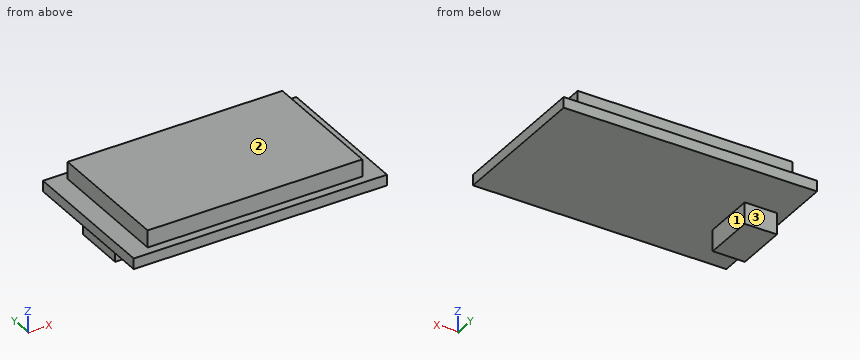
Autodesk Inventor part; units mm, degrees
ref_plane "YZ Plane" through (0, 0, 0) normal (1, 0, 0) x (0, 1, 0)
ref_plane "XZ Plane" through (0, 0, 0) normal (0, 1, 0) x (-1, 0, 0)
ref_plane "XY Plane" through (0, 0, 0) normal (0, 0, 1) x (1, 0, 0)
sketch "Sketch1" plane through (0, 0, 0) normal (0, 0, 1) x (1, 0, 0)
  line L0 (-29.5, -17) -> (29.5, -17)
  line L1 (29.5, -17) -> (29.5, 17)
  line L2 (29.5, 17) -> (-29.5, 17)
  line L3 (-29.5, 17) -> (-29.5, -17)
  line L4 (-29.5, -17) -> (29.5, 17) construction
  line L5 (29.5, -17) -> (-29.5, 17) construction
  point P0 (0, 0)
  dimension "d0" = 59
  dimension "d1" = 34
extrude "Extrusion1" add sketch "Sketch1" along normal blind 2.5
sketch "Sketch2" plane through (0, 0, 2.5) normal (0, 0, 1) x (1, 0, 0)
  line L0 (-25, -15) -> (25, -15)
  line L1 (25, -15) -> (25, 15)
  line L2 (25, 15) -> (-25, 15)
  line L3 (-25, 15) -> (-25, -15)
  line L4 (-25, -15) -> (25, 15) construction
  line L5 (25, -15) -> (-25, 15) construction
  point P0 (0, 0)
  dimension "d4" = 50
  dimension "d5" = 30
extrude "Extrusion2" add sketch "Sketch2" along normal blind 4
sketch "Sketch3" plane through (0, 0, 0) normal (0, 0, -1) x (-1, 0, 0)
  line L0 (-41.3, 0) -> (41.3, 0)
  line L1 (27, 6) -> (19.5, 6)
  line L2 (19.5, 6) -> (19.5, -6)
  line L3 (19.5, -6) -> (27, -6)
  line L4 (27, -6) -> (27, 6)
  line L5 (27, 6) -> (19.5, -6) construction
  line L6 (19.5, 6) -> (27, -6) construction
  line L7 (29.5, 17) -> (29.5, -17)
  point P0 (0, 0)
  point P1 (23.25, 0)
  dimension "d8" = 7.5
  dimension "d9" = 12
  dimension "d10" = 2.5
extrude "Extrusion3" add sketch "Sketch3" along normal blind 5
properties part number "lcdsw"
The model under review builds one solid part; all positions refer to its coordinate system, in mm. Face numbers are marked on the shaded views. A direction names the side the tool comes from. Coordinates: 2 decimals unless noted, no trailing zeros. Write each loop counter-clockwise with the first axis right and the second up, starting at its lowest first coordinate (ties: lowest second). Pieces come first, ordered by that corner, then holes. Notation, with made-up numbers: (19.5, 15.5) -> (38.5, 15.5) arc R20 cw to (38.5, 24.5) -> close; hole circle Ø7 at (53.25, -23). An arc over 180 degrees is marked (long way). One line per item, written item: value. Start each with the question number.
Q1. Add section A-A, the plane y = 3. Give the boundary of the cut face in (x, z), then the cut area to 3 significant figures.
Q2. Add section B-B, the plane x = -20.5. Give the boundary of the cut face in (y, z).
Q3. To check wall thickness, follow probe 1 along X at (y, z) = (0, -2.75); probe 2 along Z at (x, y) = (-15, -13.5); probe 3 along Y at (x, z) = (8.5, 3). State the ranges of each line that lie inside material, in increasing order.
Q4. Clearance check with flat-ended pins moving along their axes: P1, Ø10, axis at x = 21, y = 2, coming from the -Z side; P2, Ø1.5, axis at y = -0.5, z = -3, coming from the -X side; P3, Ø1.2, axis at x = 10.5, z = 5, coming from the -Y side. State where each tip first meets the part, or that it passes through.
Q5. For the marked faces 1, 2 and 3, list the 3-axis set-ups (+Z, -Z, +X, -X, +Y, -Y) from which the entire face can be reached by the end or side of a thin tool; tool diameter is ignored.
Q6. Add section C-C, the plane y = -14. Give the boundary of the cut face in (x, z), then the cut area to 4 significant figures.
Q7. Add section D-D, the plane z = 4. Give the boundary of the cut face in (x, y).
Response:
1. outline: (-29.5, 0) -> (-27, 0) -> (-27, -5) -> (-19.5, -5) -> (-19.5, 0) -> (29.5, 0) -> (29.5, 2.5) -> (25, 2.5) -> (25, 6.5) -> (-25, 6.5) -> (-25, 2.5) -> (-29.5, 2.5) -> close
1. area: 385 mm²
2. outline: (-17, 0) -> (-6, 0) -> (-6, -5) -> (6, -5) -> (6, 0) -> (17, 0) -> (17, 2.5) -> (15, 2.5) -> (15, 6.5) -> (-15, 6.5) -> (-15, 2.5) -> (-17, 2.5) -> close
3. probe 1: -27 to -19.5
3. probe 2: 0 to 6.5
3. probe 3: -15 to 15
4. P1: z = 0
4. P2: x = -27
4. P3: y = -15
5. face 1: -Z, +X, +Y, -Y
5. face 2: +Z, +X, -X, +Y, -Y
5. face 3: -Z, +X, -X, +Y
6. outline: (-29.5, 0) -> (29.5, 0) -> (29.5, 2.5) -> (25, 2.5) -> (25, 6.5) -> (-25, 6.5) -> (-25, 2.5) -> (-29.5, 2.5) -> close
6. area: 347.5 mm²
7. outline: (-25, -15) -> (25, -15) -> (25, 15) -> (-25, 15) -> close
